Verification items for the finished model (mm, model axes). A direction names the side the tool comes from. Round coordinates to 2 decimals unless told otherwise and drop trailing zeros. Loops run counter-clockwise (first coordinate to the right, second up) from the corner with the lowest first, then second, coordinate; pieces in that order, holes last. Notation, with made-up numbers: M 66.25,-12.75 L 93.25,-12.75 A27 cw 93.25,19.25 Z; hole C 15.25,69.5 d7. An arc over 180 degrees is marked long. Answer as CSV lines item,"result".
Autodesk Inventor part; units mm, degrees
ref_plane "YZ Plane" through (0, 0, 0) normal (1, 0, 0) x (0, 1, 0)
ref_plane "XZ Plane" through (0, 0, 0) normal (0, 1, 0) x (-1, 0, 0)
ref_plane "XY Plane" through (0, 0, 0) normal (0, 0, 1) x (1, 0, 0)
sketch "Sketch1" plane through (0, 0, 0) normal (1, 0, 0) x (0, 1, 0)
  line L0 (-2.5, -6.5) -> (2.5, -6.5)
  line L1 (2.5, -6.5) -> (2.5, 6.5)
  line L2 (2.5, 6.5) -> (-2.5, 6.5)
  line L3 (-2.5, 6.5) -> (-2.5, -6.5)
  line L4 (-2.5, -6.5) -> (2.5, 6.5) construction
  line L5 (2.5, -6.5) -> (-2.5, 6.5) construction
  line L6 (-10, -22.5) -> (10, -22.5)
  line L7 (10, -22.5) -> (10, 22.5)
  line L8 (10, 22.5) -> (-10, 22.5)
  line L9 (-10, 22.5) -> (-10, -22.5)
  line L10 (-10, -22.5) -> (10, 22.5) construction
  line L11 (10, -22.5) -> (-10, 22.5) construction
  circle A0 centre (2.5, 17.5) radius 1.6
  circle A1 centre (0, -17.5) radius 1.6
  point P0 (0, 0)
  dimension "d0" = 5
  dimension "d1" = 13
  dimension "d2" = 20
  dimension "d3" = 45
  dimension "d17" = 5
  dimension "d18" = 3.2
  dimension "d19" = 3.2
  dimension "d20" = 5
extrude "Extrusion1" add sketch "Sketch1" against normal blind 5 contours L9 L8 L7 L6 | A0 | A1
sketch "Sketch2" plane through (-5, 0, 0) normal (-1, 0, 0) x (0, 0, 1)
  line L0 (10, -5.5) -> (-10, -5.5)
  line L1 (-10, -5.5) -> (-10, 5.5)
  line L2 (-10, 5.5) -> (10, 5.5)
  line L3 (10, 5.5) -> (10, -5.5)
  line L4 (10, -5.5) -> (-10, 5.5) construction
  line L5 (-10, -5.5) -> (10, 5.5) construction
  line L6 (22.5, 10) -> (-22.5, 10)
  line L7 (-14, -10) -> (-14, 5.5)
  line L8 (14, 5.5) -> (14, -10)
  line L9 (12.0522, -8.6087) -> (-14, 10) construction
  line L10 (-12.0522, -8.6087) -> (14, 10) construction
  line L11 (-14, -10) -> (14, -10)
  line L12 (-14, 5.5) -> (14, 5.5)
  point P0 (0, 0)
  dimension "d6" = 20
  dimension "d7" = 11
  dimension "d27" = 4.5
  dimension "d32" = 14
  dimension "d33" = 14
extrude "Extrusion2" add sketch "Sketch2" along normal blind 27 contours L3 L12 L8 L11 L7 L1 L0
sketch "Sketch3" plane through (0, -10, -22.5) normal (0, -1, 0) x (1, 0, 0)
  point P0 (0, 22.5)
sketch "Sketch4" plane through (-32, 0, 0) normal (-1, 0, 0) x (0, 0, 1)
  line L0 (6.5, -5.5) -> (-6.5, -5.5)
  line L1 (-6.5, -5.5) -> (-6.5, 5.5)
  line L2 (-6.5, 5.5) -> (6.5, 5.5)
  line L3 (6.5, 5.5) -> (6.5, -5.5)
  line L4 (6.5, -5.5) -> (-6.5, 5.5) construction
  line L5 (-6.5, -5.5) -> (6.5, 5.5) construction
  line L6 (12.0522, -8.6087) -> (-14, 10) construction
  line L7 (-12.5, -10) -> (12.5, 10) construction
  line L8 (14, -10) -> (14, 5.5)
  line L9 (-14, -10) -> (14, -10)
  line L10 (14, -10) -> (14, 5.5)
  line L11 (14, 5.5) -> (-14, 5.5)
  line L12 (-14, 5.5) -> (-14, -10)
  point P0 (0, 0)
  point P1 (14, 10)
  dimension "d11" = 13
  dimension "d12" = 11
sketch "Sketch6" plane through (0, 0, 0) normal (1, 0, 0) x (0, 0, -1)
  circle A0 centre (17.5, 0) radius 1.6
  circle A1 centre (-17.5, 0) radius 1.6
  line L0 (22.5, -10) -> (22.5, 10)
  line L1 (-22.5, 10) -> (-22.5, -10)
  line L2 (22.5, -10) -> (14, -10)
  point P0 (0, 0)
  dimension "d21" = 3.2
  dimension "d22" = 3.2
  dimension "d23" = 5
  dimension "d24" = 5
  dimension "d41" = 10
extrude "Extrusion5" cut sketch "Sketch6" against normal blind 5
extrude "Extrusion8" add sketch "Sketch4" along normal blind 3.5 contours L3 L11 L8 L9 L12 L1 L0
sketch "Sketch8" plane through (-5, 0, 0) normal (-1, 0, 0) x (0, 0, 1)
  line L0 (-10, 5.5) -> (-10, -5.5)
  line L1 (-10, -5.5) -> (10, -5.5)
  line L2 (10, -5.5) -> (10, 6.5)
  line L3 (10, 6.5) -> (-10, 6.5)
  line L4 (-10, 6.5) -> (-10, -5.5)
  point P0 (0, 0)
  dimension "d36" = 12
extrude "Extrusion10" cut sketch "Sketch8" against normal blind 2
equation "\"BendRadius\" = Thickness"
equation "\"BendReliefWidth\" = Thickness"
equation "\"BendReliefDepth\" = 0.5 * Thickness"
equation "\"CornerReliefSize\" = 4 * Thickness"
equation "\"MinimumRemnant\" = 2 * Thickness"
equation "\"TransitionRadius\" = BendRadius"
equation "\"JacobiRadiusSize\" = Thickness"
equation "\"GapSize\" = Thickness"
properties part number "USB_housing"
1) Set-up check for faces 1 (the flat face through (-20, -2, 14)), 2 (the flat face through (-3, 3, 0)), 3 (the flat face through (-4, 6.5, 0)), 4 (the flat face through (-32, 0, -8)), 5 (the flat face through (-20, 5.5, -12)): record each of +Z, -Z, +X, -X, +Y, -Y from which the full face is reachable in a straight line by a thin tool's end or side.
Here are the results:
face 1,"+Z, -X, +Y, -Y"
face 2,"none"
face 3,"-X"
face 4,"+Y"
face 5,"+Z, -Z, -X, +Y"
2) Section check B-B (z = -0.5). Record the cut outline in (x, y).
Here are the results:
outline,"M -35.5,-10 L 0,-10 L 0,-2.5 L -3,-2.5 L -3,-5.5 L -35.5,-5.5 Z; M -5,6.5 L -3,6.5 L -3,2.5 L 0,2.5 L 0,10 L -5,10 Z"
3) Section check A-A (y = 0). Record the cut outline in (x, z).
Here are the results:
outline,"M -35.5,-14 L -5,-14 L -5,-15.9 L 0,-15.9 L 0,-6.5 L -3,-6.5 L -3,-10 L -32,-10 L -32,-6.5 L -35.5,-6.5 Z; M -35.5,6.5 L -32,6.5 L -32,10 L -3,10 L -3,6.5 L 0,6.5 L 0,15.9 L -5,15.9 L -5,14 L -35.5,14 Z; M -5,-22.5 L 0,-22.5 L 0,-19.1 L -5,-19.1 Z; M -5,19.1 L 0,19.1 L 0,22.5 L -5,22.5 Z"
4) Go/stop test with flat-tipped pins: pin 1 (3.5 mm diameter, centred on y = 0, z = -17.5, fed in from -X); pin 2 (9.5 mm diameter, centred on x = -18.5, y = 3, fed in from -Z); pin 3 (1 mm diameter, centred on y = -1, z = 8.5, fed in from +X); pin 4 (8 mm diameter, centred on x = -23.5, y = -1, fed in from +Z). Record where each tip stops, or that it passes through.
Here are the results:
pin 1,"stops at x = -5"
pin 2,"stops at z = -14"
pin 3,"stops at x = 0"
pin 4,"stops at z = 14"
5) Draft check along Z on faces 6 (the flat face through (-1, -2.5, 0)), 7 (the flat face through (-20, -2, -14)), 8 (the flat face through (-5, 7, 0)). Enter one of: +Z half, -Z half, draft (parallel to the pull), parting line (faces both ways), or undercut.
Here are the results:
face 6,"undercut"
face 7,"-Z half"
face 8,"draft"
6) Section check D-D (y = -3.25). Record the cut outline in (x, z).
Here are the results:
outline,"M -35.5,-14 L -5,-14 L -5,-22.5 L 0,-22.5 L 0,22.5 L -5,22.5 L -5,14 L -35.5,14 L -35.5,6.5 L -32,6.5 L -32,10 L -3,10 L -3,-10 L -32,-10 L -32,-6.5 L -35.5,-6.5 Z"
7) Section check C-C (x = -19). Record the cut outline in (y, z).
Here are the results:
outline,"M -10,-14 L 5.5,-14 L 5.5,-10 L -5.5,-10 L -5.5,10 L 5.5,10 L 5.5,14 L -10,14 Z"
8) Material ranges on probe 1 along Y at (x, z) = (-2.7, -17.5); probe 2 along X at (y, z) = (-3, 7.5); probe 3 along Z at (x, y) = (-12, 3.25), recorded low to high.
Here are the results:
probe 1,"y = -10 to -1.6, 1.6 to 10"
probe 2,"x = -35.5 to -32, -3 to 0"
probe 3,"z = -14 to -10, 10 to 14"
